Check sheet for the drawn part. Datum: minimum x, y, z corner. Units: mm. A direction names the side the tool comes from. Coordinates: 2 decimals unless noted, no trailing zeros. Write each loop counter-clockwise with the first axis right and the second up, starting at its lowest first coordinate (ties: lowest second). Pieces come first, ordered by that corner, then holes. Notation, with made-up numbers: M -8.75,89.5 L 17.25,89.5 A23 ccw 17.25,110.5 Z; hole C 37.5,16 d3. An arc over 180 degrees is marked long. Write item = value, one per line. Start each with the question number.
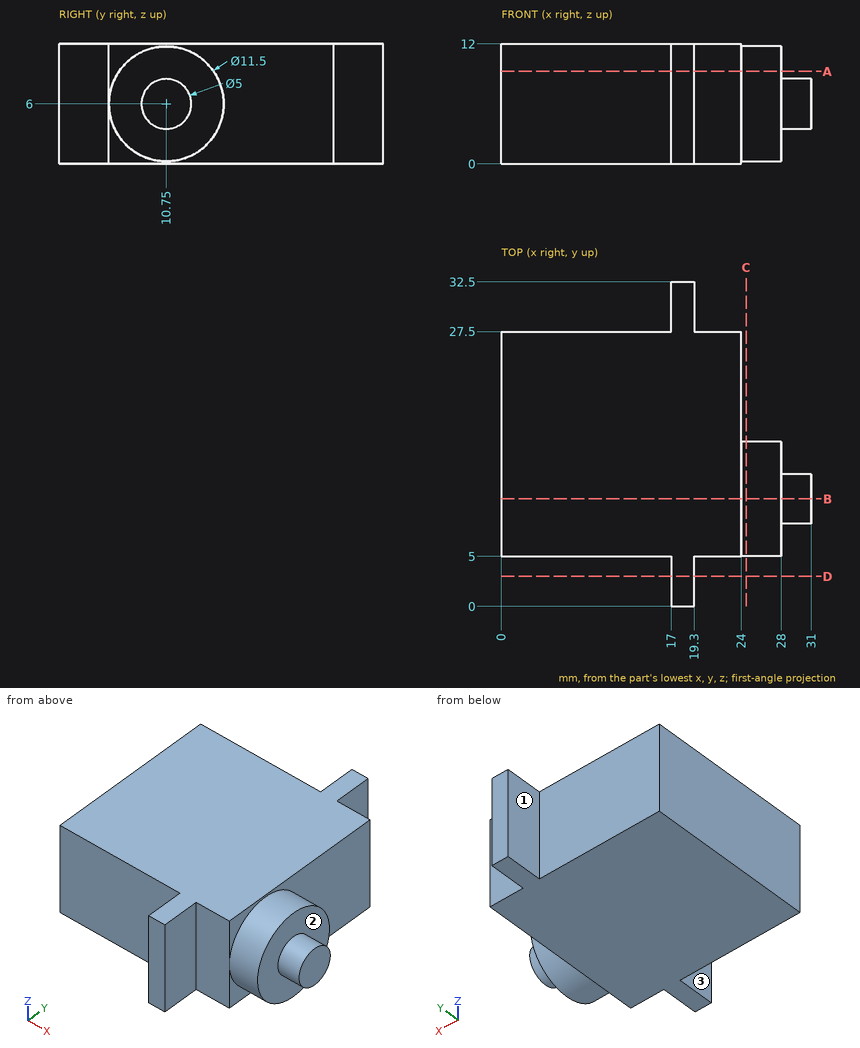
Q1. Set-up check for the marked faces 1, 2 and 3: record each of +Z, -Z, +X, -X, +Y, -Y from which the full face is reachable in a straight line by a thin tool's end or side.
Q2. Cross-section at C-C on x = 24.5. Enter the section's corners in (y, z).
Q3. Scan lines: L1, parallel to X at y = 26, z = 4.75; L2, parallel to Y at x = 14, z = 4; L3, parallel to X at y = 3, z = 1. Record each from-to range of solid material in increasing order.
Q4. Cross-section at B-B on y = 10.75. Enter the section's corners in (x, z).
Q5. Cross-section at A-A on z = 9.25. Enter the section's corners in (x, y), and give its area (3 significant figures).
Q6. Cross-section at D-D on y = 3. Enter the section's corners in (x, z).
Q7. Gauge pin test, flat ends, axial feed: pin 1 (5 mm diameter, centred on y = 25.5, z = 4.5, fed in from +X); pin 2 (4 mm diameter, centred on x = 21.5, z = 8.5, fed in from -Y); pin 3 (4 mm diameter, centred on y = 2, z = 4, fed in from +X). Record the tip position at first contact, or that the pin passes through.
Values found:
q1.face_1 = +Z, -Z, -X, +Y
q1.face_2 = +X
q1.face_3 = +Z, -Z, -X, -Y
q2.outline = C 10.75,6 d11.5
q3.L1 = 0 to 24
q3.L2 = 5 to 27.5
q3.L3 = 17 to 19.3
q4.outline = M 0,0 L 24,0 L 24,0.25 L 28,0.25 L 28,3.5 L 31,3.5 L 31,8.5 L 28,8.5 L 28,11.75 L 24,11.75 L 24,12 L 0,12 Z
q5.outline = M 0,5 L 17,5 L 17,0 L 19.3,0 L 19.3,5 L 24,5 L 24,6.01 L 28,6.01 L 28,15.49 L 24,15.49 L 24,27.5 L 19.3,27.5 L 19.3,32.5 L 17,32.5 L 17,27.5 L 0,27.5 Z
q5.area = 601 mm²
q6.outline = M 17,0 L 19.3,0 L 19.3,12 L 17,12 Z
q7.pin_1 = 24
q7.pin_2 = 5
q7.pin_3 = 19.3
